from build123d import *

# Parameters (mm, degrees)
SKETCH1_R           = 4
BOSS_EXTRUDE1_DEPTH = 2.5
SKETCH2_OUTSIDE_W   = 40.128
SKETCH2_OUTSIDE_H   = 42.604
SKETCH2_OUTSIDE_R   = 8
CUT_EXTRUDE1_DEPTH  = 6
CUT_EXTRUDE1_TAPER  = 55
CHAMFER1_SIZE       = 1


with BuildPart() as part:
    # Sketch1 → Boss-Extrude1 (new body, symmetric)
    with BuildSketch(Plane.XY):
        Polygon((-8, 4.618802154), (-8, -4.618802154), (0, -9.237604307), (8, -4.618802154), (8, 4.618802154), (0, 9.237604307), align=None)
        Circle(SKETCH1_R, mode=Mode.SUBTRACT)
    extrude(amount=BOSS_EXTRUDE1_DEPTH, both=True)

    # Sketch2 outside → Cut-Extrude1 (cut, through all)
    with BuildSketch(Plane.XY.offset(2.5)):
        Rectangle(SKETCH2_OUTSIDE_W, SKETCH2_OUTSIDE_H)
        Circle(SKETCH2_OUTSIDE_R, mode=Mode.SUBTRACT)
    cut_extrude1 = extrude(amount=-CUT_EXTRUDE1_DEPTH, taper=CUT_EXTRUDE1_TAPER, mode=Mode.SUBTRACT)

    # Mirror1: Cut-Extrude1 across plane
    add(cut_extrude1.mirror(Plane.XY), mode=Mode.SUBTRACT)

    # Chamfer1
    chamfer1_edges = [part.edges().sort_by_distance(p)[0] for p in [
        (-4, 0, -2.5),
        (-4, 0, 2.5),
    ]]
    chamfer(chamfer1_edges, length=CHAMFER1_SIZE)


solid = part.part
Build history of the part. All positions in model axes, mm. Round coordinates to 2 decimals unless told otherwise and drop trailing zeros. Order: outer loops, then holes, each group sorted by start corner. A loop starts at its lowest first (then second) coordinate and runs counter-clockwise, first axis right, second up. Notation, with made-up numbers: M 50,-19.5 L 87,-19.5 A10 ccw 87,-5.5 Z; hole C 49,22 d5. An arc over 180 degrees is marked long. Use CSV: the item, a comma, the result in double quotes. Start each with the question number.
(1) Flat gauge pins, fed straight in: P1, Ø2, axis at x = 0.5, z = 0, coming from the -Y side; P2, Ø2, axis at y = 7, z = -1, coming from the -X side. Where does each tip first touch, or does it go through?
(2) Drill centre lines: probe 1 along X at (y, z) = (-0.75, 0.5); probe 2 along X at (y, z) = (0.25, 1.6); probe 3 along Y at (x, z) = (-2, 0.35). Where is each one in solid material? Low to high.
(3) Cut at B-B on z = 2. List the corners of the cut face in (x, y), then the cut area to 3 significant figures.
(4) Cut at A-A on z = 0. List the corners of the cut face in (x, y).
(5) Mould opens along X. For faces 1 (the face through (0.02, -8.3, -2.29)), 2 (the face through (7.18, 4.17, 2.29)), 3 (the face through (-0.867, -3.905, -0.021)) say: +X half, -X half, draft (parallel to the pull), parting line (faces both ways), or undercut.
Findings:
1,P1,"stops at y = -9.24"
1,P2,"stops at x = -5.61"
2,probe 1,"x = -8 to -3.93, 3.93 to 8"
2,probe 2,"x = -8 to -4.09, 4.09 to 8"
2,probe 3,"y = -8.08 to -3.46, 3.46 to 8.08"
3,outline,"M -8,-3.45 A8.71 ccw -6.99,-5.2 L -1.01,-8.66 A8.71 ccw 1.01,-8.66 L 6.99,-5.2 A8.71 ccw 8,-3.45 L 8,3.45 A8.71 ccw 6.99,5.2 L 1.01,8.66 A8.71 ccw -1.01,8.66 L -6.99,5.2 A8.71 ccw -8,3.45 Z; hole C 0,0 d9"
3,area,"155 mm^2"
4,outline,"M -8,-4.62 L 0,-9.24 L 8,-4.62 L 8,4.62 L 0,9.24 L -8,4.62 Z; hole C 0,0 d8"
5,face 1,"parting line"
5,face 2,"+X half"
5,face 3,"undercut"
